```python
from build123d import *

# Parameters (mm, degrees)
SKETCH_1_W          = 150
SKETCH_1_H          = 20
EXTRUDE_1_DEPTH     = 10
SKETCH_2_R          = 2
CUT_EXTRUDE_1_DEPTH = 10


with BuildPart() as part:
    # 草图1 → 凸台-拉伸1 (new body)
    with BuildSketch(Plane.XY):
        Rectangle(SKETCH_1_W, SKETCH_1_H)
    extrude(amount=EXTRUDE_1_DEPTH)

    # 草图2 → 切除-拉伸1 (cut)
    with BuildSketch(Plane(origin=(0, 0, 0), x_dir=(-1, 0, 0), z_dir=(0, 0, -1))):
        with Locations((69.573976668, 0)):
            Circle(SKETCH_2_R)
        with Locations((59.573976668, 0)):
            Circle(SKETCH_2_R)
        with Locations((49.573976668, 0)):
            Circle(SKETCH_2_R)
        with Locations((39.573976668, 0)):
            Circle(SKETCH_2_R)
        with Locations((29.573976668, 0)):
            Circle(SKETCH_2_R)
        with Locations((19.573976668, 0)):
            Circle(SKETCH_2_R)
        with Locations((9.573976668, 0)):
            Circle(SKETCH_2_R)
        with Locations((-0.426023332, 0)):
            Circle(SKETCH_2_R)
        with Locations((-10.426023332, 0)):
            Circle(SKETCH_2_R)
        with Locations((-20.426023332, 0)):
            Circle(SKETCH_2_R)
        with Locations((-30.426023332, 0)):
            Circle(SKETCH_2_R)
        with Locations((-40.426023332, 0)):
            Circle(SKETCH_2_R)
        with Locations((-50.426023332, 0)):
            Circle(SKETCH_2_R)
        with Locations((-60.426023332, 0)):
            Circle(SKETCH_2_R)
    extrude(amount=-CUT_EXTRUDE_1_DEPTH, mode=Mode.SUBTRACT)


solid = part.part
```
Verification items for the finished model (mm, model axes). Give positions to 0.01 mm unless a question says otherwise; leave off trailing zeros. Put each result on its own line as item: value.
Q1. Scan line: probe 1 along Y at (x, z) = (-39, 1). Record every from-to range of solid material in increasing order. Write a range as from..to.
Result:
probe 1: -10..-1.92, 1.92..10
Q2. Depth check by flat-ended pin: P1, Ø3, axis at x = 3.5, y = 2, coming from the -Z side. Enter the tip coordinate at first touch or a pass-through.
Result:
P1: z = 0
Q3. Mould release check, pull along Y, two halves, no side actions. Record for faces 1 (the face through (-31.48, 0.6, 4.93)), 2 (the face through (-1, -10, 5)), 3 (the face through (-1, -2, 10)): released by +Y, released by -Y, zero draft, split by the parting line, or undercut.
Result:
face 1: undercut
face 2: released by -Y
face 3: zero draft
Q4. Section check A-A on z = 4.5. Count the separate pieces of the cut face and the enclosed holes in it, and give its area (3 significant figures).
Result:
separate pieces: 1
enclosed holes: 14
area: 2,820 mm2
